The model under review builds one solid part; all positions refer to its coordinate system, in mm. A direction names the side the tool comes from. Round coordinates to 2 decimals unless told otherwise and drop trailing zeros. Write each loop counter-clockwise with the first axis right and the second up, starting at its lowest first coordinate (ties: lowest second). Pieces come first, ordered by that corner, then holes.
Item 1: Add section C-C (y = -4). Give the boundary of the cut face in (x, z).
Item 2: To check wall thickness, follow L1, parallel to Z at x = 190, y = -3.5; L2, parallel to Z at x = 99.5, y = -9.25; L3, parallel to X at y = -2.75, z = 52.5. State the ranges of each line that lie inside material, in increasing order.
Item 3: Add section D-D (x = 118). Give the boundary of the cut face in (y, z), plus the area to 3 significant figures.
Item 4: Add section B-B (z = -26.5). Give the boundary of the cut face in (x, y), plus the area to 3 significant figures.
Item 5: Clearance check with flat-ended pins moving along their axes: pin 1 Ø5 at (x, y) = (-70, -3) entering from -Z; pin 2 Ø10 at (x, z) = (4, 56.5) entering from +Y; pin 3 Ø5 at (x, y) = (201, -7.5) entering from -Z; pin 4 Ø4 at (y, z) = (-7, 29.5) entering from -X. State where each tip first meets the part, or that it passes through.
Item 6: Machinability: for faces 1 (the face through (196, -5, -53.582)), 2 (the face through (178.097, -4.93, 47.291)), 3 (the face through (163.923, -5, -30)), which of the approach directions +Z, -Z, +X, -X, +Y, -Y give a long, thin tool a straight path to every point of the face, cutting with its end or side? Answer none if there is none.
Item 7: Draft analysis for pull direction Z (two halves, no side actions). For faces 4 (the face through (-199.1, -4.9, -71.8)), 5 (the face through (3, -5, 96.418)), 6 (the face through (-303.54, -4.93, -4.27)), state which applies: +Z half, -Z half, draft (parallel to the pull), parting line (faces both ways), or undercut.
Item 8: Add section A-A (x = 190). Give the boundary of the cut face in (y, z).
```python
from build123d import *

# Parameters (mm, degrees)
F0_R     = 15
F1_DEPTH = 10


with BuildPart() as f1:
    # F0 (on Front) → F1 (new body)
    with BuildSketch(Plane.XZ):
        Polygon((230, -53.581859), (230, 96.418141), (-230, 96.418141), (-344.906666, 0), (-248.488525, -114.906666), (-226.454759, -96.418141), (-170.892954, -46.418141), (-171.154469, -7.162976), (163.922563, -7.162976), (163.922563, -53.581859), align=None)
        with Locations((-288.553384, -4.930273)):
            Circle(F0_R, mode=Mode.SUBTRACT)
        with Locations((190, 56.418141)):
            Circle(F0_R, mode=Mode.SUBTRACT)
    extrude(amount=F1_DEPTH)


solid = f1.part
```
Numbers:
1. outline: (-344.91, 0) - (-248.49, -114.91) - (-226.45, -96.42) - (-170.89, -46.42) - (-171.15, -7.16) - (163.92, -7.16) - (163.92, -53.58) - (230, -53.58) - (230, 96.42) - (-230, 96.42) - close; hole circle Ø30 at (-288.55, -4.93); hole circle Ø30 at (190, 56.42)
2. L1: z = -53.58 to 41.42, 71.42 to 96.42
2. L2: z = -7.16 to 96.42
2. L3: x = -282.34 to 175.52, 204.48 to 230
3. outline: (-10, -7.16) - (0, -7.16) - (0, 96.42) - (-10, 96.42) - close
3. area: 1,040 mm2
4. outline: (-322.67, -10) - (-171.03, -10) - (-171.03, 0) - (-322.67, 0) - close; (163.92, -10) - (230, -10) - (230, 0) - (163.92, 0) - close
4. area: 2,180 mm2
5. pin 1: stops at z = -7.16
5. pin 2: stops at y = 0
5. pin 3: stops at z = -53.58
5. pin 4: stops at x = -312.13
6. face 1: -Z, +X, +Y, -Y
6. face 2: +Y, -Y
6. face 3: -Z, +Y, -Y
7. face 4: -Z half
7. face 5: +Z half
7. face 6: undercut
8. outline: (-10, -53.58) - (0, -53.58) - (0, 41.42) - (-10, 41.42) - close; (-10, 71.42) - (0, 71.42) - (0, 96.42) - (-10, 96.42) - close
